from build123d import *

# Parameters (mm, degrees)
BOSS_EXTRUDE1_DEPTH     = 4
CHAMFER1_SIZE           = 3
CUT_EXTRUDE1_DEPTH      = 34.871079109
CUT_EXTRUDE1_DEPTH_BACK = 34.871079109
SKETCH3_R               = 1.55
FILLET1_R               = 4


with BuildPart() as part:
    # Sketch1 → Boss-Extrude1 (new, symmetric)
    with BuildSketch(Plane(origin=(0, 0, 0), x_dir=(1, 0, 0), z_dir=(0, 1, 0))):
        Polygon((-25, 22.5), (25, 22.5), (25, 18.5), (15, 18.5), (15, -18.5), (25, -18.5), (25, -22.5), (-25, -22.5), (-25, -18.5), (-15, -18.5), (-15, 18.5), (-25, 18.5), align=None)
        with BuildLine():
            Line((-5, -7.5), (-5, 7.5))
            ThreePointArc((-5, 7.5), (0, 12.5), (5, 7.5))
            Line((5, 7.5), (5, -7.5))
            ThreePointArc((5, -7.5), (0, -12.5), (-5, -7.5))
        make_face(mode=Mode.SUBTRACT)
    extrude(amount=BOSS_EXTRUDE1_DEPTH, both=True)

    # Chamfer1
    chamfer1_edges = [part.edges().sort_by_distance(p)[0] for p in [
        (-15, 0, 18.5),
        (-15, 0, -18.5),
        (15, 0, -18.5),
        (15, 0, 18.5),
    ]]
    chamfer(chamfer1_edges, length=CHAMFER1_SIZE)

    # Sketch3 → Cut-Extrude1 (cut, two sides: drawn at the far end of the back side and taken through both)
    with BuildSketch(Plane.XY.offset(-CUT_EXTRUDE1_DEPTH_BACK)):
        with Locations((-21, 0)):
            Circle(SKETCH3_R)
        with Locations((21, 0)):
            Circle(SKETCH3_R)
    extrude(amount=CUT_EXTRUDE1_DEPTH + CUT_EXTRUDE1_DEPTH_BACK, mode=Mode.SUBTRACT)

    # Fillet1
    fillet1_edges = [part.edges().sort_by_distance(p)[0] for p in [
        (25, -4, 20.5),
        (-25, -4, 20.5),
        (-25, 4, 20.5),
        (25, 4, 20.5),
        (25, -4, -20.5),
        (25, 4, -20.5),
        (-25, -4, -20.5),
        (-25, 4, -20.5),
    ]]
    fillet(fillet1_edges, radius=FILLET1_R - 0.0001)  # a hair under: the kernel refuses the full size


solid = part.part
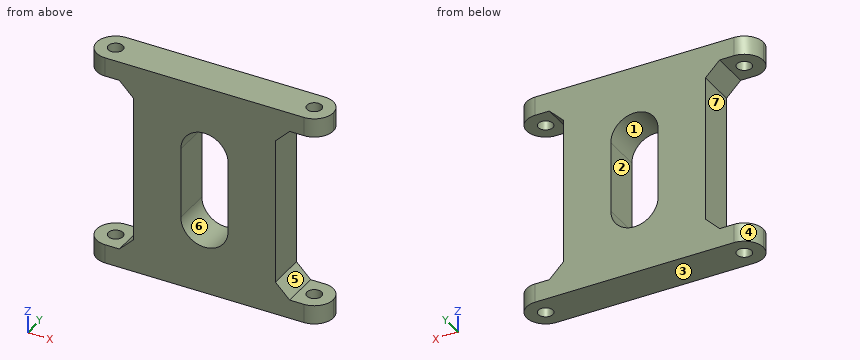
Part model, mm, in its own coordinate system. Face numbers are marked on the shaded views. A direction names the side the tool comes from. Coordinates: 2 decimals unless noted, no trailing zeros. Loops run counter-clockwise (first coordinate to the right, second up) from the corner with the lowest first, then second, coordinate; pieces in that order, holes last. Notation, with made-up numbers: (-17, 29) -> (33, 29) arc R18 cw to (33, 53) -> close; hole circle Ø11 at (-1.75, 83.5). An arc over 180 degrees is marked (long way). Use a Markdown table: item, result. Add a question column.
Item 1: Band-saw the part on C-C on y = 3.25. Write the cut outline in (x, z).
Item 2: Probe probe 1 along X at (y, z) = (0, 19.3); probe 2 along X at (y, z) = (-3, -1); probe 3 along Y at (x, z) = (-21, -21). List the from-to ranges inside material, lowest first.
Item 3: Flat gauge pins, fed straight in: P1, Ø4, axis at y = -0.5, z = -3, coming from the -X side; P2, Ø3, axis at y = -1, z = -2.5, coming from the +X side. Where does each tip first touch, or does it go through?
Item 4: Band-saw the part on A-A on z = -10.5. Write the cut outline in (x, y), plus the area to 3 significant figures.
Item 5: Which spindle directions (+Z, -Z, +X, -X, +Y, -Y) get a long thin tool onto all of the face, cutting with end or side? Do the marked faces 5, 6 and 7. Say none if no direction does.
Item 6: Band-saw the part on B-B on x = 0. Write the cut outline in (y, z), plus the area to 3 significant figures.
Item 7: Pull direction Z, two halves, no side cores. Call the marked faces 1, 2, 3 and 4: +Z half, -Z half, draft (parallel to the pull), parting line (faces both ways), or undercut.
Geometry says:
| question | item | result |
|---|---|---|
| 1 | outline | (-23.33, -22.5) -> (23.33, -22.5) -> (23.33, -18.5) -> (18, -18.5) -> (15, -15.5) -> (15, 15.5) -> (18, 18.5) -> (23.33, 18.5) -> (23.33, 22.5) -> (-23.33, 22.5) -> (-23.33, 18.5) -> (-18, 18.5) -> (-15, 15.5) -> (-15, -15.5) -> (-18, -18.5) -> (-23.33, -18.5) -> close; hole (-5, -7.5) arc R5 ccw to (5, -7.5) -> (5, 7.5) arc R5 ccw to (-5, 7.5) -> close |
| 2 | probe 1 | -25 to -22.55, -19.45 to 19.45, 22.55 to 25 |
| 2 | probe 2 | -15 to -5, 5 to 15 |
| 2 | probe 3 | -4 to -1.55, 1.55 to 4 |
| 3 | P1 | x = -15 |
| 3 | P2 | x = 15 |
| 4 | outline | (-15, -4) -> (-4, -4) -> (-4, 4) -> (-15, 4) -> close; (4, -4) -> (15, -4) -> (15, 4) -> (4, 4) -> close |
| 4 | area | 176 mm² |
| 5 | face 5 | +X, +Y, -Y |
| 5 | face 6 | +Y, -Y |
| 5 | face 7 | -X, +Y, -Y |
| 6 | outline | (-4, -22.5) -> (4, -22.5) -> (4, -12.5) -> (-4, -12.5) -> close; (-4, 12.5) -> (4, 12.5) -> (4, 22.5) -> (-4, 22.5) -> close |
| 6 | area | 160 mm² |
| 7 | face 1 | undercut |
| 7 | face 2 | undercut |
| 7 | face 3 | -Z half |
| 7 | face 4 | draft |
